Work out the finished part from the listing and answer in its coordinate system (mm). Face numbers are marked on the shaded views. A direction names the side the tool comes from. Give positions to 0.01 mm unless a question says otherwise; leave off trailing zeros. Loops run counter-clockwise (first coordinate to the right, second up) from the corner with the lowest first, then second, coordinate; pieces in that order, holes last.
```python
from build123d import *

# Parameters (mm, degrees)
BOSS_EXTRUDE1_DEPTH = 3.175
SKETCH2_W           = 39.37
SKETCH2_H           = 3.175
BOSS_EXTRUDE2_DEPTH = 33.02
SKETCH3_W           = 39.37
SKETCH3_H           = 8.89
SKETCH3_H_2         = 3.175
BOSS_EXTRUDE3_DEPTH = 3.175
SKETCH4_W           = 8.89
SKETCH4_H           = 33.02
BOSS_EXTRUDE4_DEPTH = 3.1242
RIB1_REACH          = 45.93
SKETCH6_WALL_W      = 122.696858414
SKETCH6_WALL_H      = 2.54
FILLET1_R           = 1.27


with BuildPart() as part:
    # Sketch1 → Boss-Extrude1 (new body)
    with BuildSketch(Plane(origin=(0, 0, 0), x_dir=(1, 0, 0), z_dir=(0, 1, 0))):
        Polygon((-12.065, 15.24), (-19.685, 12.838646177), (-19.685, 0), (19.685, 0), (19.685, 12.838646177), (12.065, 15.24), align=None)
        with BuildLine():
            ThreePointArc((-14.295, 9.2075), (-10.795, 12.7075), (-7.295, 9.2075))
            Line((-7.295, 9.2075), (-7.295, 6.0325))
            ThreePointArc((-7.295, 6.0325), (-10.795, 2.5325), (-14.295, 6.0325))
            Line((-14.295, 6.0325), (-14.295, 9.2075))
        make_face(mode=Mode.SUBTRACT)
        with BuildLine():
            Line((7.295, 6.0325), (7.295, 9.2075))
            ThreePointArc((7.295, 9.2075), (10.795, 12.7075), (14.295, 9.2075))
            Line((14.295, 9.2075), (14.295, 6.0325))
            ThreePointArc((14.295, 6.0325), (10.795, 2.5325), (7.295, 6.0325))
        make_face(mode=Mode.SUBTRACT)
    extrude(amount=BOSS_EXTRUDE1_DEPTH)

    # Sketch2 → Boss-Extrude2 (add)
    with BuildSketch(Plane(origin=(0, 0, 0), x_dir=(1, 0, 0), z_dir=(0, 1, 0))):
        with Locations((0, -1.5875)):
            Rectangle(SKETCH2_W, SKETCH2_H)
    extrude(amount=BOSS_EXTRUDE2_DEPTH)

    # Sketch3 → Boss-Extrude3 (add)
    with BuildSketch(Plane(origin=(0, 33.02, 0), x_dir=(1, 0, 0), z_dir=(0, 1, 0))):
        with Locations((0, -7.62)):
            Rectangle(SKETCH3_W, SKETCH3_H)
        with Locations((0, -1.5875)):
            Rectangle(SKETCH3_W, SKETCH3_H_2)
    extrude(amount=BOSS_EXTRUDE3_DEPTH)

    # Sketch4 → Boss-Extrude4 (add)
    with BuildSketch(Plane(origin=(19.685, 0, 0), x_dir=(0, 0, -1), z_dir=(1, 0, 0))):
        with Locations((-7.62, 16.51)):
            Rectangle(SKETCH4_W, SKETCH4_H)
    extrude(amount=-BOSS_EXTRUDE4_DEPTH)

    # Sketch6 wall → Rib1 (add, up to next)
    with BuildSketch(Plane(origin=(0, 18.152288456, -6.726767741), x_dir=(0, -0.912217845065, -0.409705507828), z_dir=(0, 0.409705507828, -0.912217845065)), mode=Mode.PRIVATE) as rib1_sk1:
        Rectangle(SKETCH6_WALL_W, SKETCH6_WALL_H)
    rib1_tool1 = extrude(rib1_sk1.sketch, amount=-RIB1_REACH, mode=Mode.PRIVATE) - part.part
    add(rib1_tool1.solids().sort_by_distance((0, 18.152288456, -6.726767741))[0])

    # Fillet1
    fillet1_edges = [part.edges().sort_by_distance(p)[0] for p in [
        (-1.27, 3.175, -6.726767741),
        (1.27, 3.175, -6.726767741),
        (-1.27, 18.152288456, 0),
        (19.685, 3.175, -6.419323088),
        (15.875, 3.175, -14.039323088),
        (0, 3.175, -15.24),
        (-15.875, 3.175, -14.039323088),
        (-19.685, 3.175, -6.419323088),
        (-10.4775, 3.175, 0),
        (-19.685, 19.685, 0),
        (19.685, 19.685, 0),
        (19.685, 36.195, 6.0325),
        (0, 36.195, 0),
        (-19.685, 36.195, 6.0325),
        (10.4775, 3.175, 0),
        (0, 33.129576912, 0),
        (1.27, 18.152288456, 0),
    ]]
    fillet(fillet1_edges, radius=FILLET1_R)


solid = part.part
```
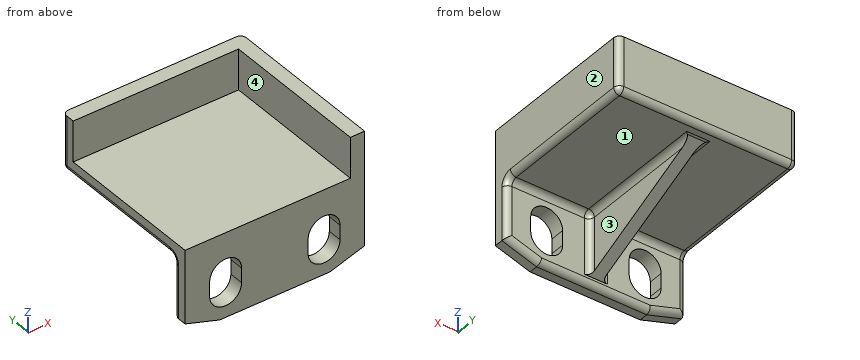
Q1. Section C-C on z = 4.5 is taken. Give the vertices of the cut face in (x, y) (3 decimals), plus the area to 3 significant figures.
Q2. Section D-D on x = 6 is taken. Give the vertices of the cut face in (y, z) (3 decimals), plus the area to 3 significant figures.
Q3. Section B-B on x = 10 is taken. Give the vertices of the cut face in (y, z) (3 decimals), plus the area to 3 significant figures.
Q4. Consider line 1 along Z through (x, y) = (-2.5, 32) (3 decimals); line 2 along Z through (x, y) = (-5.5, 34) (3 decimals); line 3 along Y through (x, z) = (15.5, 9.25) (3 decimals). Determine where each line is inside the solid, lowest interval first.
Q5. Which of the six approach directions +Z, -Z, +X, -X, +Y, -Y give full straight-line access (tool end or side, diameter ignored) to the marked faces 1, 2, 3 and 4?
Q6. Given pin 1 (1.6 mm diameter, centred on y = 2, z = -7, fed in from +X) (3 decimals); pin 2 (10 mm diameter, centred on x = -7, y = 17.5, fed in from +Z) (3 decimals); pin 3 (6 mm diameter, centred on y = 20, z = -4.5, fed in from -X); pin 4 (1 mm diameter, centred on y = 16, z = -1.5, fed in from +X), each flat-ended and moving along its own axis, determine where each tip first touches the part or whether it passes through.
Q7. Section A-A on z = -11 is taken. Give the vertices of the cut face in (x, y) (3 decimals).
Check result:
1. outline: (-19.685, 33.02) - (16.561, 33.02) - (16.561, 0) - (19.685, 0) - (19.685, 34.925) arc R1.27 ccw to (18.415, 36.195) - (-18.415, 36.195) arc R1.27 ccw to (-19.685, 34.925) - close
1. area: 227 mm2
2. outline: (0, -15.24) - (1.905, -15.24) arc R1.27 ccw to (3.175, -13.97) - (3.175, -1.27) arc R1.27 cw to (4.445, 0) - (34.925, 0) arc R1.27 ccw to (36.195, 1.27) - (36.195, 12.065) - (33.02, 12.065) - (33.02, 3.175) - (0, 3.175) - close
2. area: 191 mm2
3. outline: (0, -15.24) - (1.905, -15.24) arc R1.27 ccw to (3.175, -13.97) - (3.175, -12.616) - (0, -12.616) - close; (0, -2.624) - (3.175, -2.624) - (3.175, -1.27) arc R1.27 cw to (4.445, 0) - (34.925, 0) arc R1.27 ccw to (36.195, 1.27) - (36.195, 12.065) - (33.02, 12.065) - (33.02, 3.175) - (0, 3.175) - close
3. area: 159 mm2
4. line 1: z = -0.001 to 3.175
4. line 2: z = 0 to 12.065
4. line 3: y = 33.02 to 36.195
5. face 1: -Z, +Y
5. face 2: +Z, -Z, +X, +Y, -Y
5. face 3: -Z, +X, +Y
5. face 4: +Z, -X, -Y
6. pin 1: stops at x = 19.685
6. pin 2: stops at z = 3.175
6. pin 3: stops at x = -1.27
6. pin 4: stops at x = 1.3
7. outline: (-19.685, 0) - (-13.801, 0) - (-13.801, 3.175) - (-18.415, 3.175) arc R1.27 ccw to (-19.685, 1.905) - close; (-7.789, 0) - (7.789, 0) - (7.789, 3.175) - (2.54, 3.175) arc R1.27 cw to (1.27, 4.445) - (1.27, 8.638) - (-1.27, 8.638) - (-1.27, 4.445) arc R1.27 cw to (-2.54, 3.175) - (-7.789, 3.175) - close; (13.801, 0) - (19.685, 0) - (19.685, 1.905) arc R1.27 ccw to (18.415, 3.175) - (13.801, 3.175) - close
